from build123d import *

# Parameters (mm, degrees)
F0_W     = 50
F0_H     = 50
F1_DEPTH = 8
F2_R     = 6.15
F3_DEPTH = 2
F4_R     = 1.75
F5_DEPTH = 6.001


with BuildPart() as f1:
    # F0 (on Top) → F1 (new body)
    with BuildSketch(Plane.XY):
        Rectangle(F0_W, F0_H)
    extrude(amount=-F1_DEPTH)

    # F2 (on face) → F3 (cut)
    with BuildSketch(Plane.XY):
        Circle(F2_R)
    extrude(amount=-F3_DEPTH, mode=Mode.SUBTRACT)

    # F4 (on face) → F5 (cut, through all)
    with BuildSketch(Plane.XY.offset(-2)):
        Circle(F4_R)
    extrude(amount=-F5_DEPTH, mode=Mode.SUBTRACT)


solid = f1.part
Can you work these out from the model? Positions are in its coordinate system, mm. A direction names the side the tool comes from. Give positions to 0.01 mm unless a question says otherwise; leave off trailing zeros. Order: outer loops, then holes, each group sorted by start corner. A loop starts at its lowest first (then second) coordinate and runs counter-clockwise, first axis right, second up. Notation, with made-up numbers: M -18,-26 L 30,-26 A20 cw 30,-1 Z; hole C -39.75,-20.75 d10. An arc over 180 degrees is marked long. One line per item, written item: value.
Item 1: Please list where these lines run through material, in increasing order: line 1 (Y direction, x = 0, z = -1.25); line 2 (Y direction, x = 0, z = -5.3); line 3 (Z direction, x = -5, y = -0.5).
Verdict:
line 1: -25 to -6.15, 6.15 to 25
line 2: -25 to -1.75, 1.75 to 25
line 3: -8 to -2
Item 2: If we section it at C-C on z = -1: Write out the boundary of the cut face in (x, y).
Verdict:
outline: M -25,-25 L 25,-25 L 25,25 L -25,25 Z; hole C 0,0 d12.3
Item 3: If we mould it in two halves opening along Y, with no side actions, what happens to faces 1 (the face through (0, 6, -8)), 2 (the face through (0, 25, -4)), 3 (the face through (0, -25, -4)), 4 (the face through (1.617, -0.67, -4.958))? For each: pulls with the +Y half, pulls with the -Y half, needs draft (parallel to the pull), parting line crosses it, or undercut.
Verdict:
face 1: needs draft
face 2: pulls with the +Y half
face 3: pulls with the -Y half
face 4: undercut
Item 4: For faces 5 (the face through (-1.333, -6.004, -0.986)), 6 (the face through (-25, 0, -4)), which set-ups out of +Z, -Z, +X, -X, +Y, -Y let a thin tool reach every point of the face, with its end or its side?
Verdict:
face 5: +Z
face 6: +Z, -Z, -X, +Y, -Y
Item 5: If we section it at A-A on y = 0: Write out the boundary of the cut face in (x, z).
Verdict:
outline: M -25,-8 L -1.75,-8 L -1.75,-2 L -6.15,-2 L -6.15,0 L -25,0 Z; M 1.75,-8 L 25,-8 L 25,0 L 6.15,0 L 6.15,-2 L 1.75,-2 Z
Item 6: For pin 1 (10 mm diameter, centred on x = 0, y = 0, fed in from +Z), with a flat end and sliding along its axis, tell me the tip position at first contact or that it passes through.
Verdict:
pin 1: z = -2
